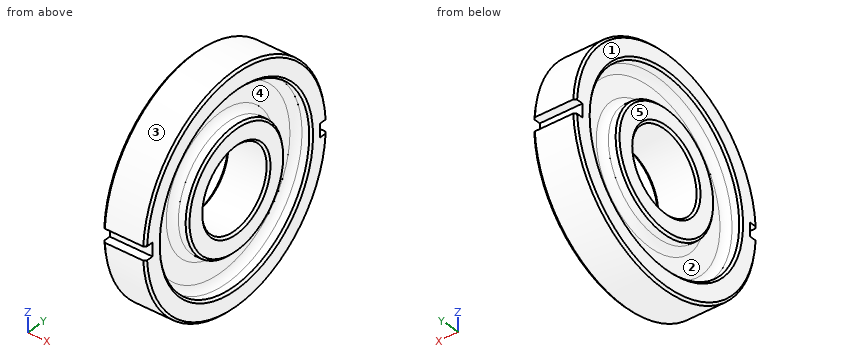
Autodesk Inventor part; units mm, degrees
ref_plane "YZ Plane" through (0, 0, 0) normal (1, 0, 0) x (0, 1, 0)
ref_plane "XZ Plane" through (0, 0, 0) normal (0, 1, 0) x (-1, 0, 0)
ref_plane "XY Plane" through (0, 0, 0) normal (0, 0, 1) x (1, 0, 0)
sketch "Эскиз1" plane through (0, 0, 0) normal (0, 0, 1) x (1, 0, 0)
  line L0 (0, 0) -> (28.5418, 0) construction
  line L1 (0, 30) -> (32, 30)
  line L2 (32, 30) -> (32, 45)
  line L3 (32, 45) -> (25, 45)
  line L4 (20, 50) -> (20, 64.408)
  line L5 (25, 69.408) -> (32, 69.408)
  line L6 (32, 69.408) -> (32, 84.358)
  line L7 (32, 84.358) -> (9.7618, 84.358)
  line L8 (9.7618, 84.358) -> (0, 84.358)
  line L9 (0, 84.358) -> (0, 69.408)
  line L10 (0, 69.408) -> (7, 69.408)
  line L11 (12, 64.408) -> (12, 50)
  line L12 (7, 45) -> (0, 45)
  line L13 (0, 45) -> (0, 30)
  arc A0 (7, 45) -> (12, 50) centre (7, 50) ccw
  arc A1 (12, 64.408) -> (7, 69.408) centre (7, 64.408) ccw
  arc A2 (25, 69.408) -> (20, 64.408) centre (25, 64.408) ccw
  arc A3 (20, 50) -> (25, 45) centre (25, 50) ccw
  line L14 (-7.6009, 77.608) -> (48.6633, 77.608)
  point P0 (11, 45)
  point P1 (12, 46)
  point P2 (21, 45)
  point P3 (20, 46)
  point P4 (12, 75.15)
  point P5 (11, 69.408)
  point P6 (21, 69.408)
  point P7 (20, 75.15)
  dimension "d0" = 32
  dimension "d3" = 32
  dimension "d7" = 60
  dimension "d8" = 168.716
  dimension "d11" = 90
  dimension "d13" = 90
  dimension "d15" = 8
  dimension "d16" = 12
  dimension "d23" = 5
  dimension "d24" = 155.216
  dimension "d25" = 8.2
  dimension "d26" = 8.2
revolve "Вращение1" add sketch "Эскиз1" angle 360 about axis through (0, 0, 0) along (1, 0, 0)
chamfer "Фаска1" distance 1.6 angle 45 8 edges at (0, -84.358, 0) (0, -69.408, 0) (32, -84.358, 0) (32, -69.408, 0) (32, -30, 0) (0, -30, 0) (32, -45, 0) (0, -45, 0)
sketch "Эскиз3" plane through (0, 0, 0) normal (0, 0, 1) x (1, 0, 0)
  line L0 (1.6, 84.358) -> (30.4, 84.358)
  line L1 (7, 69.408) -> (1.6, 69.408)
  line L2 (0, -82.758) -> (0, 82.758)
  line L3 (32, 82.758) -> (32, -82.758)
  line L4 (1.6, 84.358) -> (37.8818, 84.358)
  line L5 (37.8818, 84.358) -> (37.8818, 77.608)
  line L6 (37.8818, 77.608) -> (1.6, 77.608)
  line L7 (1.6, 77.608) -> (-1.0807, 77.608)
  line L8 (-1.0807, 77.608) -> (-1.0807, 84.358)
  line L9 (-1.0807, 84.358) -> (2.0712, 84.358)
  line L10 (0, 0) -> (69.5045, 0)
  line L11 (1.6, -84.358) -> (30.4, -84.358)
  line L12 (7, -69.408) -> (1.6, -69.408)
  line L13 (1.6, -84.358) -> (37.8818, -84.358)
  line L14 (37.8818, -84.358) -> (37.8818, -77.608)
  line L15 (37.8818, -77.608) -> (1.6, -77.608)
  line L16 (1.6, -77.608) -> (-1.0807, -77.608)
  line L17 (-1.0807, -77.608) -> (-1.0807, -84.358)
  line L18 (-1.0807, -84.358) -> (2.0712, -84.358)
  dimension "d20" = 77.608
extrude "Выдавливание1" cut sketch "Эскиз3" against normal mid plane 10 contours L0 L4 L5 L6 L7 L8 L9 | L16 L15 L14 L13 L11 L18 L17
equation "\"d16\" = -0.5 * d15 + 0.5 * d0"
properties part number "Тихоходное колесо"
Geometry check sheet. Reference: the model listing, model coordinates, mm. Face numbers are marked on the shaded views. A direction names the side the tool comes from. Coordinates: 2 decimals unless noted, no trailing zeros. Loops run counter-clockwise (first coordinate to the right, second up) from the corner with the lowest first, then second, coordinate; pieces in that order, holes last. Notation, with made-up numbers: (21.25, 21.5) -> (60.25, 21.5) arc R23 ccw to (60.25, 38.5) -> close; hole circle Ø1 at (28.5, 36). An arc over 180 degrees is marked (long way). Put each result on its own line as item: value.
1) Cross-section at A-A on x = 27.5. Record the boundary of the cut face in (y, z).
Result set:
outline: (-84.21, -5) arc R84.36 ccw to (84.21, -5) -> (77.61, -5) -> (77.61, 5) -> (84.21, 5) arc R84.36 ccw to (-84.21, 5) -> (-77.61, 5) -> (-77.61, -5) -> close; circle Ø90 at (0, 0); hole circle Ø138.82 at (0, 0); hole circle Ø60 at (0, 0)
2) Cross-section at B-B on x = 15. Record the boundary of the cut face in (y, z), plus the area to 3 significant figures.
Result set:
outline: (-84.21, -5) arc R84.36 ccw to (84.21, -5) -> (77.61, -5) -> (77.61, 5) -> (84.21, 5) arc R84.36 ccw to (-84.21, 5) -> (-77.61, 5) -> (-77.61, -5) -> close; hole circle Ø60 at (0, 0)
area: 19,400 mm^2
3) Tool access check on the marked faces 4 and 5. Record the directions out of +Z, -Z, +X, -X, +Y, -Y that give a thin tool (end or side, any length) a straight path to the whole face; none if there is none.
Result set:
face 4: +X
face 5: +Z, -Z, -X, +Y, -Y
4) Thickness scan on line 1 (Z direction, x = 28.55, y = 0); line 2 (Y direction, x = 6.5, z = -13.5); line 3 (Z direction, x = 22, y = 0). Record the ranges inside material, lowest first.
Result set:
line 1: z = -84.36 to -69.41, -45 to -30, 30 to 45, 69.41 to 84.36
line 2: y = -83.27 to -68.08, -42.93 to -26.79, 26.79 to 42.93, 68.08 to 83.27
line 3: z = -84.36 to -68.41, -46 to -30, 30 to 46, 68.41 to 84.36
5) Release check for a two-part mould opening along Y. For the marked faces 1, 2 and 3 record: released by +Y, released by -Y, zero draft, split by the parting line, or undercut.
Result set:
face 1: zero draft
face 2: undercut
face 3: split by the parting line
6) Gauge pin test, flat ends, axial feed: pin 1 Ø7.5 at (x, y) = (19.5, 82) entering from -Z; pin 2 Ø6 at (x, z) = (6.5, 54.5) entering from +Y; pin 3 Ø3 at (x, z) = (19.5, 1) entering from +Y. Record the tip position at first contact, or that the pin passes through.
Result set:
pin 1: stops at z = -31.52
pin 2: stops at y = 66.81
pin 3: stops at y = 77.61
